CAD build for the part. Positions are in the model's coordinates, mm. A direction names the side the tool comes from. Round coordinates to 2 decimals unless told otherwise and drop trailing zeros. Order: outer loops, then holes, each group sorted by start corner. A loop starts at its lowest first (then second) coordinate and runs counter-clockwise, first axis right, second up. Notation, with made-up numbers: (39.5, 23) - (63.5, 23) arc R24 cw to (63.5, 57) - close; hole circle Ø1 at (-30.75, 18.25). An arc over 180 degrees is marked (long way). Use one line per item in the form item = value. Start each with the question number.
from build123d import *

# Parameters (mm, degrees)
SKETCH1_W            = 169.5
SKETCH1_H            = 38
BOSS_EXTRUDE1_DEPTH  = 3
SKETCH12_W           = 40
SKETCH12_H           = 3
BOSS_EXTRUDE3_DEPTH  = 38
SKETCH16_W           = 37
SKETCH16_H           = 3
BOSS_EXTRUDE4_DEPTH  = 38
SKETCH18_W           = 37
SKETCH18_H           = 163.5
BOSS_EXTRUDE5_DEPTH  = 3
FILLET1_R            = 2
FILLET2_R            = 2
FILLET3_R            = 2
FILLET4_R            = 2
SKETCH37_W           = 165.5
SKETCH37_H           = 25
BOSS_EXTRUDE12_DEPTH = 3
SKETCH40_W           = 25
SKETCH40_H           = 25
BOSS_EXTRUDE13_DEPTH = 3
FILLET11_R           = 25
SKETCH41_W           = 25
SKETCH41_H           = 25
BOSS_EXTRUDE14_DEPTH = 3
FILLET12_R           = 25
CUT_EXTRUDE19_DEPTH  = 10
SKETCH62_R           = 4
CUT_EXTRUDE23_DEPTH  = 10
SKETCH66_R           = 0.875
CUT_EXTRUDE24_DEPTH  = 10
SKETCH63_R           = 1
CUT_EXTRUDE26_DEPTH  = 10
SKETCH19_W           = 37
SKETCH19_H           = 163.5
BOSS_EXTRUDE16_DEPTH = 3
SKETCH123_R          = 13.061371159
CUT_EXTRUDE30_DEPTH  = 3
SKETCH125_R          = 13
CUT_EXTRUDE31_DEPTH  = 3
SKETCH126_R          = 13
CUT_EXTRUDE32_DEPTH  = 3
SKETCH67_R           = 12
CUT_EXTRUDE33_DEPTH  = 3
SKETCH118_R          = 12
CUT_EXTRUDE34_DEPTH  = 3


with BuildPart() as part:
    # Sketch1 → Boss-Extrude1 (new body)
    with BuildSketch(Plane(origin=(0, 0, 0), x_dir=(0, 0, -1), z_dir=(1, 0, 0))):
        with Locations((84.75, 19)):
            Rectangle(SKETCH1_W, SKETCH1_H)
    extrude(amount=BOSS_EXTRUDE1_DEPTH)

    # Sketch12 → Boss-Extrude3 (add)
    with BuildSketch(Plane(origin=(0, 0, -169.5), x_dir=(1, 0, 0), z_dir=(0, 1, 0))):
        with Locations((20, -1.5)):
            Rectangle(SKETCH12_W, SKETCH12_H)
    extrude(amount=BOSS_EXTRUDE3_DEPTH)

    # Sketch16 → Boss-Extrude4 (add)
    with BuildSketch(Plane(origin=(3, 0, 0), x_dir=(1, 0, 0), z_dir=(0, 1, 0))):
        with Locations((18.5, 1.5)):
            Rectangle(SKETCH16_W, SKETCH16_H)
    extrude(amount=BOSS_EXTRUDE4_DEPTH)

    # Sketch18 → Boss-Extrude5 (add)
    with BuildSketch(Plane(origin=(0, 38, 0), x_dir=(1, 0, 0), z_dir=(0, 1, 0))):
        with Locations((21.5, 84.75)):
            Rectangle(SKETCH18_W, SKETCH18_H)
    extrude(amount=-BOSS_EXTRUDE5_DEPTH)

    # Fillet1
    fillet1_edges = [part.edges().sort_by_distance(p)[0] for p in [
        (20, 0, 0),
    ]]
    fillet(fillet1_edges, radius=FILLET1_R)

    # Fillet2
    fillet2_edges = [part.edges().sort_by_distance(p)[0] for p in [
        (20, 38, 0),
    ]]
    fillet(fillet2_edges, radius=FILLET2_R)

    # Fillet3
    fillet3_edges = [part.edges().sort_by_distance(p)[0] for p in [
        (20, 38, -169.5),
    ]]
    fillet(fillet3_edges, radius=FILLET3_R)

    # Fillet4
    fillet4_edges = [part.edges().sort_by_distance(p)[0] for p in [
        (20, 0, -169.5),
    ]]
    fillet(fillet4_edges, radius=FILLET4_R)

    # Sketch37 → Boss-Extrude12 (add)
    with BuildSketch(Plane.ZY):
        with Locations((-84.75, 50.5)):
            Rectangle(SKETCH37_W, SKETCH37_H)
    extrude(amount=-BOSS_EXTRUDE12_DEPTH)

    # Sketch40 → Boss-Extrude13 (add)
    with BuildSketch(Plane(origin=(0, 0, -167.5), x_dir=(-1, 0, 0), z_dir=(0, 0, -1))):
        with Locations((-15.5, 50.5)):
            Rectangle(SKETCH40_W, SKETCH40_H)
    extrude(amount=-BOSS_EXTRUDE13_DEPTH)

    # Fillet11
    fillet11_edges = [part.edges().sort_by_distance(p)[0] for p in [
        (28, 63, -166),
    ]]
    fillet(fillet11_edges, radius=FILLET11_R - 0.0001)  # a hair under: the kernel refuses the full size

    # Sketch41 → Boss-Extrude14 (add)
    with BuildSketch(Plane.XY.offset(-2)):
        with Locations((15.5, 50.5)):
            Rectangle(SKETCH41_W, SKETCH41_H)
    extrude(amount=-BOSS_EXTRUDE14_DEPTH)

    # Fillet12
    fillet12_edges = [part.edges().sort_by_distance(p)[0] for p in [
        (28, 63, -3.5),
    ]]
    fillet(fillet12_edges, radius=FILLET12_R - 0.0001)  # a hair under: the kernel refuses the full size

    # Sketch57 → Cut-Extrude19 (cut)
    with BuildSketch(Plane(origin=(3, 0, 0), x_dir=(0, 0, -1), z_dir=(1, 0, 0))):
        with BuildLine():
            Line((11.018645082, 52.249341523), (74.018645082, 52.249341523))
            ThreePointArc((74.018645082, 52.249341523), (76.518645082, 49.749341523), (74.018645082, 47.249341523))
            Line((74.018645082, 47.249341523), (11.018645082, 47.249341523))
            ThreePointArc((11.018645082, 47.249341523), (8.518645082, 49.749341523), (11.018645082, 52.249341523))
        make_face()
        with BuildLine():
            Line((158.918944647, 47.24934152), (95.918944647, 47.24934152))
            ThreePointArc((95.918944647, 47.24934152), (93.418944647, 49.74934152), (95.918944647, 52.24934152))
            Line((95.918944647, 52.24934152), (158.918944647, 52.24934152))
            ThreePointArc((158.918944647, 52.24934152), (161.418944647, 49.74934152), (158.918944647, 47.24934152))
        make_face()
    extrude(amount=-CUT_EXTRUDE19_DEPTH, mode=Mode.SUBTRACT)

    # Sketch62 → Cut-Extrude23 (cut)
    with BuildSketch(Plane(origin=(0, 38, 0), x_dir=(1, 0, 0), z_dir=(0, 1, 0))):
        with Locations(Location((25.649526178, 84.75, 0), (0, 0, 270))):
            Circle(SKETCH62_R)
    extrude(amount=-CUT_EXTRUDE23_DEPTH, mode=Mode.SUBTRACT)

    # Sketch66 → Cut-Extrude24 (cut)
    with BuildSketch(Plane(origin=(0, 38, 0), x_dir=(1, 0, 0), z_dir=(0, 1, 0))):
        with Locations(Location((25.649526178, 102.75, 0), (0, 0, 270))):
            Circle(SKETCH66_R)
    extrude(amount=-CUT_EXTRUDE24_DEPTH, mode=Mode.SUBTRACT)

    # Sketch63 → Cut-Extrude26 (cut)
    with BuildSketch(Plane(origin=(0, 38, 0), x_dir=(1, 0, 0), z_dir=(0, 1, 0))):
        with Locations(Location((25.649526178, 66.75, 0), (0, 0, 270))):
            Circle(SKETCH63_R)
    extrude(amount=-CUT_EXTRUDE26_DEPTH, mode=Mode.SUBTRACT)

    # Sketch19 → Boss-Extrude16 (add)
    with BuildSketch(Plane(origin=(0, 0, 0), x_dir=(-1, 0, 0), z_dir=(0, -1, 0))):
        with Locations((-21.5, 84.75)):
            Rectangle(SKETCH19_W, SKETCH19_H)
    extrude(amount=-BOSS_EXTRUDE16_DEPTH)

    # Sketch123 → Cut-Extrude30 (cut)
    with BuildSketch(Plane.ZY):
        with Locations((-144.75, 20.2809694)):
            Circle(SKETCH123_R)
    extrude(amount=-CUT_EXTRUDE30_DEPTH, mode=Mode.SUBTRACT)

    # Sketch125 → Cut-Extrude31 (cut)
    with BuildSketch(Plane.ZY):
        with Locations((-24.75, 20.2809694)):
            Circle(SKETCH125_R)
    extrude(amount=-CUT_EXTRUDE31_DEPTH, mode=Mode.SUBTRACT)

    # Sketch126 → Cut-Extrude32 (cut)
    with BuildSketch(Plane.ZY):
        with Locations((-114.75, 20.2809694)):
            Circle(SKETCH126_R)
    extrude(amount=-CUT_EXTRUDE32_DEPTH, mode=Mode.SUBTRACT)

    # Sketch67 → Cut-Extrude33 (cut)
    with BuildSketch(Plane.ZY):
        with Locations((-84.75, 20.2809694)):
            Circle(SKETCH67_R)
    extrude(amount=-CUT_EXTRUDE33_DEPTH, mode=Mode.SUBTRACT)

    # Sketch118 → Cut-Extrude34 (cut)
    with BuildSketch(Plane.ZY):
        with Locations((-54.75, 20.2809694)):
            Circle(SKETCH118_R)
    extrude(amount=-CUT_EXTRUDE34_DEPTH, mode=Mode.SUBTRACT)


solid = part.part
(1) Which spindle directions (+Z, -Z, +X, -X, +Y, -Y) get a long thin tool onto all of the face, cutting with end or side? Do faces 1 (the cylindrical face through (1.52, 49.8, -161.42)), 2 (the flat face through (1, 63, -84)), 3 (the flat face through (22, 3, -86)), 4 (the cylindrical face through (24.118, 36.521, -81.055)), 5 (the flat face through (0, 39, -86)). Say none if no direction does.
(2) Mould opens along Y. For faces 6 (the flat face through (20, 0, -86)), 7 (the flat face through (21, 19, -166.5)), 8 (the flat face through (21, 38, -86)), 9 (the flat face through (11, 48, -2)) say: pulls with the +Y half, pulls with the -Y half, needs draft (parallel to the pull), parting line crosses it, or undercut.
(3) Flat gauge pins, fed straight in: P1, Ø1.5, axis at x = 5, y = 44.5, coming from the -Z side; P2, Ø18.5, axis at x = 28.5, z = -50, coming from the +Y side; P3, Ø2, axis at y = 41, z = -131, coming from the +X side. Where does each tip first touch, or does it go through?
(4) Wall check: line 1 (Z direction, x = 34, y = 17); line 2 (Y direction, x = 1.8, z = -84.75); line 3 (Y direction, x = 4.5, z = -8). Give the ranges that are in metal, low to high. Write a range as [from, to].
(5) Slice it at C-C (y = 26). Give the cut face in (x, z).
(6) Slice it at D-D (z = -54.75). Give the cut face in (x, y).
(7) Slice it at A-A (z = -144.75). Give the cut face in (x, y).
(8) Slice it at B-B (x = 35.5). Give the cut face in (y, z), and give its area (3 significant figures).
Results list:
q1.face_1 = +X, -X
q1.face_2 = +Z, -Z, +X, -X, +Y
q1.face_3 = +X
q1.face_4 = +Y
q1.face_5 = +Z, -Z, -X, +Y, -Y
q2.face_6 = pulls with the -Y half
q2.face_7 = undercut
q2.face_8 = pulls with the +Y half
q2.face_9 = needs draft
q3.P1 = -167.5
q3.P2 = 38
q3.P3 = 3
q4.line_1 = [-169.5, -166.5], [-3, 0]
q4.line_2 = [0, 8.28], [32.28, 63]
q4.line_3 = [0, 3], [35, 38]
q5.outline = (0, -169.5) - (40, -169.5) - (40, -166.5) - (3, -166.5) - (3, -156.49) - (0, -156.49) - close; (0, -133.01) - (3, -133.01) - (3, -126.42) - (0, -126.42) - close; (0, -103.08) - (3, -103.08) - (3, -95.3) - (0, -95.3) - close; (0, -74.2) - (3, -74.2) - (3, -65.3) - (0, -65.3) - close; (0, -44.2) - (3, -44.2) - (3, -36.42) - (0, -36.42) - close; (0, -13.08) - (3, -13.08) - (3, -3) - (40, -3) - (40, 0) - (0, 0) - close
q6.outline = (0, 0) - (40, 0) - (40, 3) - (3, 3) - (3, 8.28) - (0, 8.28) - close; (0, 32.28) - (3, 32.28) - (3, 35) - (40, 35) - (40, 38) - (3, 38) - (3, 47.25) - (0, 47.25) - close; (0, 52.25) - (3, 52.25) - (3, 63) - (0, 63) - close
q7.outline = (0, 0) - (40, 0) - (40, 3) - (3, 3) - (3, 7.22) - (0, 7.22) - close; (0, 33.34) - (3, 33.34) - (3, 35) - (40, 35) - (40, 38) - (3, 38) - (3, 47.25) - (0, 47.25) - close; (0, 52.25) - (3, 52.25) - (3, 63) - (0, 63) - close
q8.outline = (0, -167.5) arc R2 ccw to (2, -169.5) - (36, -169.5) arc R2 ccw to (38, -167.5) - (38, -2) arc R2 ccw to (36, 0) - (2, 0) arc R2 ccw to (0, -2) - close; hole (3, -166.5) - (35, -166.5) - (35, -3) - (3, -3) - close
q8.area = 1,210 mm²
